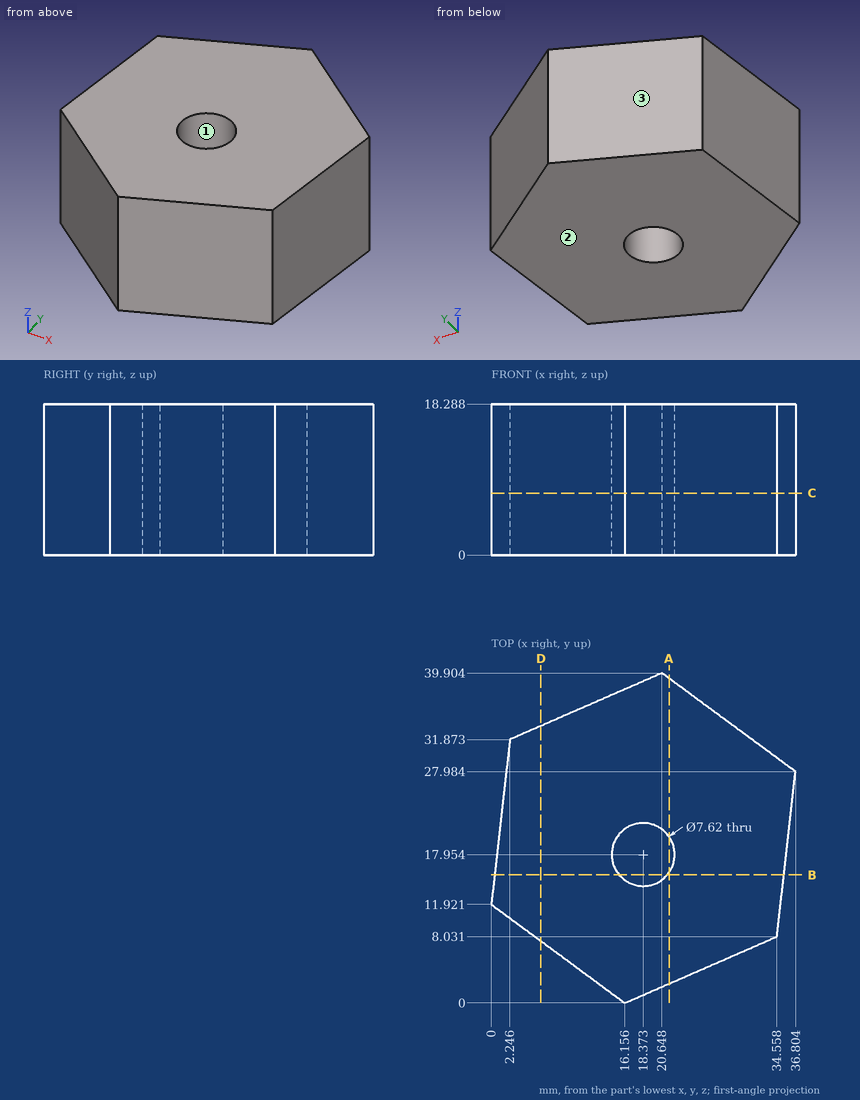
The drawing under review shows one solid part. Ordinate dimensions are in mm from its lowest x, y, z. Round coordinates to 2 decimals unless told otherwise and drop trailing zeros. Loops run counter-clockwise (first coordinate to the right, second up) from the corner with the lowest first, then second, coordinate; pieces in that order, holes last. Notation, with made-up numbers: (-32, 33.25) - (-22, 33.25) arc R22 cw to (-22, 72.25) - close; hole circle Ø9 at (-14, 34). An arc over 180 degrees is marked (long way). One line per item, written item: value. Start each with the question number.
1) Consider section D-D on x = 6. Give the boundary of the cut face in (y, z).
2) Consider section B-B on y = 15.5. Give the boundary of the cut face in (x, z).
3) Consider section A-A on x = 21.5. Give the boundary of the cut face in (y, z) (1 decimal), then the cut area to 3 significant figures.
4) To check wall thickness, follow L1, parallel to Y at x = 16, z = 12.5 (1 decimal); L2, parallel to Y at x = 19, z = 10 (1 decimal); L3, parallel to Y at x = 10, z = 6.75 (1 decimal). State the ranges of each line that lie inside material, in increasing order. Write a range as from..to.
5) Consider section C-C on z = 7.5. Give the boundary of the cut face in (x, y) (1 decimal), then the cut area to 3 significant figures.
6) Draft analysis for pull direction Y (two halves, no side actions). For the marked faces 1, 2 and 3, state which applies: +Y half, -Y half, draft (parallel to the pull), parting line (faces both ways), or undercut.
7) Insertion check: pin 1 Ø8 at (y, z) = (22.5, 5.5) entering from -X; pin 2 Ø5 at (x, z) = (13.5, 6) entering from +Y (1 decimal); pin 3 Ø3 at (y, z) = (33.5, 3) entering from +X; pin 4 Ø4.5 at (x, y) = (18.37, 17.95) entering from -Z. Each pin has a flat end and moves straight along its axis. Give the tip position at first contact, or say it passes through.
Reported:
1. outline: (7.49, 0) - (33.51, 0) - (33.51, 18.29) - (7.49, 18.29) - close
2. outline: (0.4, 0) - (15.46, 0) - (15.46, 18.29) - (0.4, 18.29) - close; (21.29, 0) - (35.4, 0) - (35.4, 18.29) - (21.29, 18.29) - close
3. outline: (2.3, 0) - (15.8, 0) - (15.8, 18.3) - (2.3, 18.3) - close; (20.1, 0) - (39.3, 0) - (39.3, 18.3) - (20.1, 18.3) - close
3. area: 596 mm^2
4. L1: y = 0.1..15, 20.9..37.9
4. L2: y = 1.2..14.2, 21.7..39.2
4. L3: y = 4.5..35.3
5. outline: (0, 11.9) - (16.2, 0) - (34.6, 8) - (36.8, 28) - (20.6, 39.9) - (2.2, 31.9) - close; hole circle Ø7.6 at (18.4, 18)
5. area: 1,000 mm^2
6. face 1: undercut
6. face 2: draft
6. face 3: +Y half
7. pin 1: stops at x = 0.74
7. pin 2: stops at y = 37.9
7. pin 3: stops at x = 31.36
7. pin 4: passes through
